Here's how the part is built. I have some questions about the finished solid (model axes, mm). A direction names the side the tool comes from. Round coordinates to 2 decimals unless told otherwise and drop trailing zeros. Write each loop counter-clockwise with the first axis right and the second up, starting at its lowest first coordinate (ties: lowest second). Pieces come first, ordered by that corner, then holes. Notation, with made-up numbers: M -1,18.5 L 22,18.5 A34 ccw 22,48.5 Z; hole C 77,64.5 d10. An arc over 180 degrees is marked long. Write item = value, one per line. Start each with the question number.
(1) I want a section at A-A (y = 5). List the corners of the cut face in (x, z) for me.
(2) Will these pins go through, and if not, where does the flat tip stop? pin 1 Ø10 at (x, z) = (41.5, 13.5) entering from +Y; pin 2 Ø0.9 at (y, z) = (11, -14) entering from +X.
(3) I need wall thicknesses on line 1 along X through (y, z) = (4.75, 24); line 2 along Z through (x, y) = (47.5, 3); line 3 along X through (y, z) = (2, 29). Which ranges of each line are inside material? Lowest first, please.
(4) On a 3-axis mill with a long thin cutter (end or side, diameter ignored), from which of +Z, -Z, +X, -X, +Y, -Y can I reach the whole of each face in a straight line? I mean faces 1 (the flat face through (43, 10, -1)), 2 (the flat face through (-25, 11, 1)), 3 (the cylindrical face through (48, 5, -30)), 4 (the flat face through (0, 3, 1)). Say none if no direction works.
(5) If we mould it in two halves opening along X, with no side actions, what happens to faces 5 (the cylindrical face through (-48, 5, -30)), 6 (the flat face through (60, 5, 0)), 7 (the cylindrical face through (-56.39, 4.93, 32.58)), 8 (the flat face through (-42, 10, -1))? For each: released by +X, released by -X, zero draft, split by the parting line, or undercut.
(6) I want a section at B-B (z = -4.5). List the corners of the cut face in (x, y) for me, and give its area (3 significant figures).
(7) I want a section at C-C (x = 16). List the corners of the cut face in (y, z) for me, and give its area (3 significant figures).
```python
from build123d import *

# Parameters (mm, degrees)
BOSS_EXTRUDE1_DEPTH = 10
SKETCH2_W           = 50
SKETCH2_H           = 72
BOSS_EXTRUDE2_DEPTH = 3
SKETCH3_W           = 50
SKETCH3_H           = 72
CUT_EXTRUDE1_DEPTH  = 3
SKETCH4_R           = 6
CUT_EXTRUDE3_DEPTH  = 49


with BuildPart() as part:
    # Sketch1 → Boss-Extrude1 (new body)
    with BuildSketch(Plane(origin=(0, 0, 0), x_dir=(1, 0, 0), z_dir=(0, 1, 0))):
        with BuildLine():
            Line((-48, 36), (48, 36))
            ThreePointArc((48, 36), (56.485281374, 32.485281374), (60, 24))
            Line((60, 24), (60, -24))
            ThreePointArc((60, -24), (56.485281374, -32.485281374), (48, -36))
            Line((48, -36), (-48, -36))
            ThreePointArc((-48, -36), (-56.485281374, -32.485281374), (-60, -24))
            Line((-60, -24), (-60, 24))
            ThreePointArc((-60, 24), (-56.485281374, 32.485281374), (-48, 36))
        make_face()
    extrude(amount=BOSS_EXTRUDE1_DEPTH)

    # Sketch2 → Boss-Extrude2 (add)
    with BuildSketch(Plane(origin=(0, 10, 0), x_dir=(1, 0, 0), z_dir=(0, 1, 0))):
        Rectangle(SKETCH2_W, SKETCH2_H)
    extrude(amount=BOSS_EXTRUDE2_DEPTH)

    # Sketch3 → Cut-Extrude1 (cut)
    with BuildSketch(Plane.XZ):
        Rectangle(SKETCH3_W, SKETCH3_H)
    extrude(amount=-CUT_EXTRUDE1_DEPTH, mode=Mode.SUBTRACT)

    # Sketch4 → Cut-Extrude3 (cut)
    with BuildSketch(Plane(origin=(0, 10, 0), x_dir=(1, 0, 0), z_dir=(0, 1, 0))):
        with Locations(Location((48, 24, 0), (0, 0, 270))):
            Circle(SKETCH4_R)
        with Locations(Location((48, -24, 0), (0, 0, 270))):
            Circle(SKETCH4_R)
        with Locations(Location((-48, -24, 0), (0, 0, 270))):
            Circle(SKETCH4_R)
        with Locations(Location((-48, 24, 0), (0, 0, 270))):
            Circle(SKETCH4_R)
    extrude(amount=-CUT_EXTRUDE3_DEPTH, mode=Mode.SUBTRACT)


solid = part.part
```
Returned:
q1.outline = M -60,-24 A12 ccw -48,-36 L 48,-36 A12 ccw 60,-24 L 60,24 A12 ccw 48,36 L -48,36 A12 ccw -60,24 Z; hole C -48,-24 d12; hole C -48,24 d12; hole C 48,-24 d12; hole C 48,24 d12
q2.pin_1 = 10
q2.pin_2 = 25
q3.line_1 = -60 to -54, -42 to 42, 54 to 60
q3.line_2 = -36 to -29.98, -18.02 to 18.02, 29.98 to 36
q3.line_3 = -58.91 to -51.32, -44.68 to -25, 25 to 44.68, 51.32 to 58.91
q4.face_1 = +Z, -Z, +X, +Y
q4.face_2 = +Z, -Z, -X, +Y
q4.face_3 = +Y, -Y
q4.face_4 = +Z, -Z, -Y
q5.face_5 = undercut
q5.face_6 = released by +X
q5.face_7 = released by -X
q5.face_8 = zero draft
q6.outline = M -60,0 L -25,0 L -25,3 L 25,3 L 25,0 L 60,0 L 60,10 L 25,10 L 25,13 L -25,13 L -25,10 L -60,10 Z
q6.area = 1,200 mm²
q7.outline = M 3,-36 L 13,-36 L 13,36 L 3,36 Z
q7.area = 720 mm²
